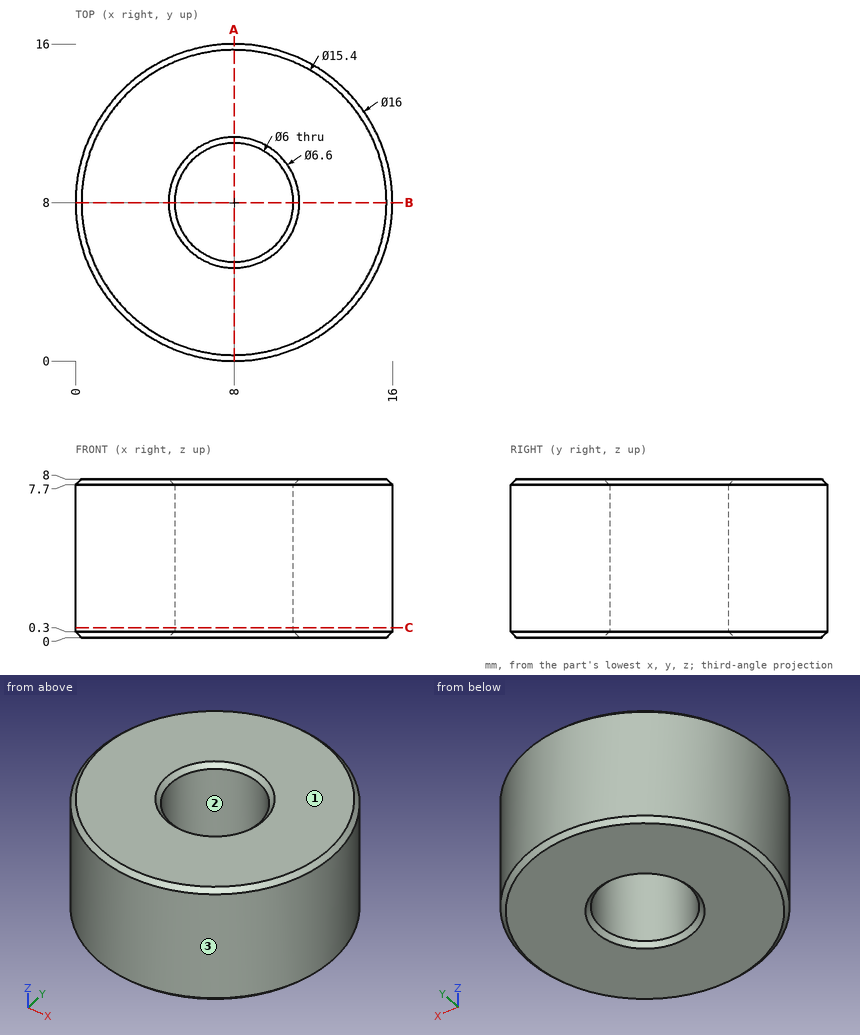
Print and shaded views of the part. All mm, measured from the part's lowest x, y and z. Round coordinates to 2 decimals unless told otherwise and drop trailing zeros. Write each loop counter-clockwise with the first axis right and the second up, starting at its lowest first coordinate (ties: lowest second). Pieces come first, ordered by that corner, then holes. Notation, with made-up numbers: (-5.5, 50) - (-1.5, 50) arc R21 cw to (-1.5, 64) - close; hole circle Ø1 at (75.5, 16.5). An arc over 180 degrees is marked (long way). Use CSV: the item, a comma, the result in double quotes. Start each with the question number.
Item 1: Two-plate mould, pull along Y, no slides. Class the marked faces 1, 2 and 3: released by +Y, released by -Y, zero draft, split by the parting line, or undercut.
Item 2: Drill centre lines: L1, parallel to Y at x = 8, z = 5.5; L2, parallel to Y at x = 5.5, z = 3.5; L3, parallel to X at y = 7.5, z = 1.5. Where is each one in solid material? Low to high. Write a range as [from, to].
Item 3: Pin check, flat tips, straight feed: P1, Ø1.5, axis at x = 13.5, z = 2, coming from the +Y side; P2, Ø3, axis at y = 3.5, z = 1, coming from the -X side; P3, Ø3, axis at x = 10.5, z = 4, coming from the +Y side. Stop position of each tip, or through.
Item 4: Band-saw the part on A-A (x = 8). Write the cut outline in (y, z).
Item 5: Band-saw the part on C-C (z = 0.5). Write the cut outline in (x, y).
Checked values:
1,face 1,"zero draft"
1,face 2,"undercut"
1,face 3,"split by the parting line"
2,L1,"y = [0, 5], [11, 16]"
2,L2,"y = [0.4, 6.34], [9.66, 15.6]"
2,L3,"x = [0.02, 5.04], [10.96, 15.98]"
3,P1,"stops at y = 14.44"
3,P2,"stops at x = 0.58"
3,P3,"stops at y = 15.94"
4,outline,"(0, 0.3) - (0.3, 0) - (4.7, 0) - (5, 0.3) - (5, 7.7) - (4.7, 8) - (0.3, 8) - (0, 7.7) - close; (11, 0.3) - (11.3, 0) - (15.7, 0) - (16, 0.3) - (16, 7.7) - (15.7, 8) - (11.3, 8) - (11, 7.7) - close"
5,outline,"circle Ø16 at (8, 8); hole circle Ø6 at (8, 8)"
